Can you work these out from the model? Positions are in its coordinate system, mm. A direction names the side the tool comes from. Give positions to 0.01 mm unless a question says otherwise; leave off trailing zeros. Write each loop counter-clockwise with the first axis right and the second up, starting at its lowest first coordinate (ties: lowest second). Pieces come first, ordered by that corner, then holes.
1. On a 3-axis mill with a long thin cutter (end or side, diameter ignored), from which of +Z, -Z, +X, -X, +Y, -Y can I reach the whole of each face in a straight line? I mean faces 4 (the flat face through (236, -28, 3.571)), 5 (the flat face through (19, -28, 3.571)), 6 (the flat face through (128, -28, 15.875)), 7 (the flat face through (209.2, -28.17, 6.17)), 8 (the flat face through (126, 0, 13)). Say none if no direction works.
2. Suppose I cut it at D-D (x = 19). Please give me the cut outline in (y, z).
3. Suppose I cut it at C-C (z = 7.75). Please give me the cut outline in (x, y).
4. Suppose I cut it at A-A (y = -44.45). Please give me the cut outline in (x, z) (3 decimals), and give its area (3 significant figures).
5. If I drill on probe 1 along X at (y, z) = (-44.45, 15.15); probe 2 along X at (y, z) = (-44.45, 13.2); probe 3 along Z at (x, y) = (10, -23.5), over which ranges is the centre line in solid material (lowest first)?
6. I'm going to push flat-ended pins straight in: pin 1 (6 mm diameter, centred on y = -44, z = 10, fed in from -X); pin 2 (1.5 mm diameter, centred on y = -44.5, z = 4.5, fed in from -X); pin 3 (8 mm diameter, centred on x = 216, y = -44, fed in from +Z). Where does each tip first touch, or does it pass through?
7. Thinking about a two-plate mould opening in Y: for faces 1 (the cylindrical face through (177.424, -44.677, 13.998)), 2 (the flat face through (234, -28, 0)), 3 (the flat face through (126, -57.15, 13)), which applies, pulls with the +Y half, pulls with the -Y half, needs draft (parallel to the pull), parting line crosses it, or undercut?
8. Suppose I cut it at B-B (y = -6). Please give me the cut outline in (x, z) (3 decimals), and give its area (3 significant figures).
```python
from build123d import *

# Parameters (mm, degrees)
F1_DEPTH = 57.15
F2_R     = 5.1562
F3_DEPTH = 25.4


with BuildPart() as f1:
    # F0 (on Front) → F1 (new body)
    with BuildSketch(Plane.XZ):
        Polygon((0, 3.57124), (0, 0), (38.627791, 0), (50.8, 12.172209), (51.9684, 12.172209), (127, 12.172209), (203.2, 12.172209), (215.372209, 0), (254, 0), (254, 3.57124), (216.851466, 3.57124), (204.547706, 15.875), (49.452294, 15.875), (37.148534, 3.57124), align=None)
    extrude(amount=F1_DEPTH)

    # F2 (on face) → F3 (cut)
    with BuildSketch(Plane(origin=(0, 0, 0), x_dir=(1, 0, 0), z_dir=(0, 0, -1))):
        with Locations((71.4502, 44.45)):
            Circle(F2_R)
        with Locations((182.5752, 44.45)):
            Circle(F2_R)
    extrude(amount=-F3_DEPTH, mode=Mode.SUBTRACT)


solid = f1.part
```
Checks:
1. face 4: +Z, +X, +Y, -Y
1. face 5: +Z, -X, +Y, -Y
1. face 6: +Z, +X, -X, +Y, -Y
1. face 7: -Z, +Y, -Y
1. face 8: +Z, -Z, +X, -X, +Y
2. outline: (-57.15, 0) - (0, 0) - (0, 3.57) - (-57.15, 3.57) - close
3. outline: (41.33, -57.15) - (46.38, -57.15) - (46.38, 0) - (41.33, 0) - close; (207.62, -57.15) - (212.67, -57.15) - (212.67, 0) - (207.62, 0) - close
4. outline: (0, 0) - (38.628, 0) - (50.8, 12.172) - (66.294, 12.172) - (66.294, 15.875) - (49.452, 15.875) - (37.149, 3.571) - (0, 3.571) - close; (76.606, 12.172) - (177.419, 12.172) - (177.419, 15.875) - (76.606, 15.875) - close; (187.731, 12.172) - (203.2, 12.172) - (215.372, 0) - (254, 0) - (254, 3.571) - (216.851, 3.571) - (204.548, 15.875) - (187.731, 15.875) - close
4. area: 887 mm2
5. probe 1: x = 48.73 to 66.29, 76.61 to 177.42, 187.73 to 205.27
5. probe 2: x = 46.78 to 66.29, 76.61 to 177.42, 187.73 to 207.22
5. probe 3: z = 0 to 3.57
6. pin 1: stops at x = 40.58
6. pin 2: stops at x = 37.33
6. pin 3: stops at z = 8.42
7. face 1: undercut
7. face 2: needs draft
7. face 3: pulls with the -Y half
8. outline: (0, 0) - (38.628, 0) - (50.8, 12.172) - (203.2, 12.172) - (215.372, 0) - (254, 0) - (254, 3.571) - (216.851, 3.571) - (204.548, 15.875) - (49.452, 15.875) - (37.149, 3.571) - (0, 3.571) - close
8. area: 964 mm2
